Check sheet for the modelled part. Datum: model origin and axes. Units: mm. A direction names the side the tool comes from. Give positions to 0.01 mm unless a question says otherwise; leave off trailing zeros. Order: outer loops, then holes, each group sorted by start corner. A loop starts at its lowest first (then second) coordinate and runs counter-clockwise, first axis right, second up. Notation, with made-up numbers: (4.25, 29) -> (15.25, 29) arc R38 cw to (15.25, 67) -> close; hole circle Ø9 at (75.5, -25.5). An arc over 180 degrees is marked (long way). Write each question's results on one line, items separated by ' | '.
from build123d import *

# Parameters (mm, degrees)
F0_W        = 19.1829744726
F0_H        = 41.2798188627
F1_DEPTH    = 8.636
F2_W        = 65.804887563
F2_H        = 25.253537111
F2_R        = 7.2247324081
F3_DEPTH    = 7.874
F4_W        = 40.3897017241
F4_H        = 12.0197124779
F5_DEPTH    = 25.4
F6_T4_DEPTH = 221.0461057398


# Not quite as in the source:
# - a fillet or chamfer that OpenCascade refuses, or shapes differently, is made with other operations: its cross-section is extruded or revolved along the edge and cut away or added


with BuildPart() as f1:
    # F0 (on Right) → F1 (new body)
    with BuildSketch(Plane.YZ):
        with Locations((9.5914872363, 8.6201969534)):
            Rectangle(F0_W, F0_H)
        Polygon((35.4520790279, 5.2206832916), (19.1829744726, 29.2601063848), (19.1829744726, -12.0197124779), (35.4520790279, -12.0197124779), align=None)
    extrude(amount=F1_DEPTH)

    # F2 (on face) → F3 (join)
    with BuildSketch(Plane.XZ):
        Polygon((-16.9975720346, -12.0197124779), (8.636, -12.0197124779), (8.636, 36.0591337085), (-16.9975720346, 36.0591337085), (-16.9975720346, 13.2338246331), align=None)
        with Locations((-49.9000158161, 0.6070560776)):
            Rectangle(F2_W, F2_H)
        with Locations((-67.2618225217, 0)):
            Circle(F2_R, mode=Mode.SUBTRACT)
        Polygon((-82.8024595976, 13.2338246331), (-16.9975720346, 13.2338246331), (-16.9975720346, 36.0591337085), align=None)
    extrude(amount=F3_DEPTH)

    # F4 (on face) → F5 (join)
    with BuildSketch(Plane(origin=(0, 0, 0), x_dir=(-1, 0, 0), z_dir=(0, 1, 0))):
        with Locations((20.194850862, -6.009856239)):
            Rectangle(F4_W, F4_H)
    extrude(amount=F5_DEPTH)

    # F6: chamfer of 40.64 on 1 edges, made by hand


with BuildPart() as f6_tool2:
    # F6_s3 → F6_t4 (new body)
    with BuildSketch(Plane.XY.offset(-116.5329091089)):
        Polygon((-40.3897017241, -15.24), (0.2502982759, 25.4), (-40.3897017241, 25.4), align=None)
    extrude(amount=F6_T4_DEPTH)

    split(bisect_by=Plane.XZ, keep=Keep.BOTTOM)

    split(bisect_by=Plane.YZ, keep=Keep.BOTTOM)


with BuildPart() as f1_1:
    add(f1.part)

    # F6_t1: cut F6_tool2
    add(f6_tool2.part, mode=Mode.SUBTRACT)


solid = f1_1.part
1. Section check A-A on y = -5. Record the cut outline in (x, z), then the cut area to 3 significant figures.
Verdict:
outline: (-82.8, -12.02) -> (8.64, -12.02) -> (8.64, 36.06) -> (-17, 36.06) -> (-82.8, 13.23) -> close; hole circle Ø14.45 at (-67.26, 0) | area: 3,480 mm^2
2. Access from +Z, -Z, +X, -X, +Y, -Y to the whole of each face (thin tool, end or side, straight path). Record for faces 4 (the flat face through (-82.802, -4, 0)), 5 (the flat face through (4, 9, 29.26)), 6 (the flat face through (-10, 10, 0)).
Verdict:
face 4: +Z, -Z, -X, +Y, -Y | face 5: +Z, +X, -X, +Y | face 6: +Z, -X, +Y
3. Material ranges on probe 1 along Y at (x, z) = (-56, 3.5); probe 2 along X at (y, z) = (26.5, 11); probe 3 along Z at (x, y) = (1, 14.5), recorded low to high. Write a range as from..to.
Verdict:
probe 1: y = -7.87..0 | probe 2: x = 0..8.64 | probe 3: z = -12.02..29.26
4. Section check C-C on x = -70. Record the cut outline in (y, z), then the cut area to 3 significant figures.
Verdict:
outline: (-7.87, -12.02) -> (0, -12.02) -> (0, -6.69) -> (-7.87, -6.69) -> close; (-7.87, 6.69) -> (0, 6.69) -> (0, 17.67) -> (-7.87, 17.67) -> close | area: 129 mm^2
5. Section check B-B on z = -3. Record the cut outline in (x, y), then the cut area to 3 significant figures.
Verdict:
outline: (-82.8, -7.87) -> (-73.83, -7.87) -> (-73.83, 0) -> (-82.8, 0) -> close; (-60.69, -7.87) -> (8.64, -7.87) -> (8.64, 35.45) -> (0, 35.45) -> (0, 25.15) -> (-25.15, 0) -> (-60.69, 0) -> close | area: 1,240 mm^2
6. Mould release check, pull along X, two halves, no side actions. Record for faces 1 (the flat face through (0, 17, 9)), 2 (the cylindrical face through (-74.48, -3.88, 0.32)), 3 (the flat face through (-16, 4, -12.02)): +X half, -X half, draft (parallel to the pull), parting line (faces both ways), or undercut.
Verdict:
face 1: -X half | face 2: undercut | face 3: draft
7. Gauge pin test, flat ends, axial feed: pin 1 Ø2 at (y, z) = (14, 18) entering from -X; pin 2 Ø4.5 at (x, y) = (6, 5.5) entering from +Z; pin 3 Ø3 at (y, z) = (10, -1) entering from -X. Record the tip position at first contact, or that the pin passes through.
Verdict:
pin 1: stops at x = 0 | pin 2: stops at z = 29.26 | pin 3: stops at x = -16.65
8. Section check D-D on y = 11. Record the cut outline in (x, z), then the cut area to 3 significant figures.
Verdict:
outline: (-14.15, -12.02) -> (8.64, -12.02) -> (8.64, 29.26) -> (0, 29.26) -> (0, 0) -> (-14.15, 0) -> close | area: 527 mm^2
